Autodesk Inventor part; units mm, degrees
ref_plane "YZ Plane" through (0, 0, 0) normal (1, 0, 0) x (0, 1, 0)
ref_plane "XZ Plane" through (0, 0, 0) normal (0, 1, 0) x (-1, 0, 0)
ref_plane "XY Plane" through (0, 0, 0) normal (0, 0, 1) x (1, 0, 0)
sketch "Sketch1" plane through (0, 0, 0) normal (0, 1, 0) x (-1, 0, 0)
  line L0 (82.5, 55) -> (-82.5, 55)
  line L1 (-82.5, 55) -> (-82.5, -55)
  line L2 (-82.5, -55) -> (82.5, -55)
  line L3 (82.5, -55) -> (82.5, 55)
  line L4 (82.5, 55) -> (-82.5, -55) construction
  line L5 (-82.5, 55) -> (82.5, -55) construction
  point P0 (0, 0)
  dimension "d0" = 165
  dimension "d1" = 110
extrude "Extrusion1" add sketch "Sketch1" along normal blind 15
sketch "Sketch3" plane through (0, 15, 0) normal (0, 1, 0) x (1, 0, 0)
  line L0 (82.5, -55) -> (82.5, 55)
  line L1 (-82.5, -35.5) -> (82.5, -35.5)
  line L2 (82.5, -35.5) -> (82.5, 35.5)
  line L3 (82.5, 35.5) -> (-82.5, 35.5)
  line L4 (-82.5, 35.5) -> (-82.5, -35.5)
  line L5 (-82.5, -35.5) -> (82.5, 35.5) construction
  line L6 (82.5, -35.5) -> (-82.5, 35.5) construction
  point P0 (0, 0)
  dimension "d8" = 71
extrude "Extrusion3" cut sketch "Sketch3" against normal blind 5
sketch "Sketch4" plane through (0, 15, 0) normal (0, 1, 0) x (1, 0, 0)
  circle A0 centre (-67.5, -45) radius 4
  line L0 (-82.5, -55) -> (82.5, -55)
  line L1 (-82.5, -35.5) -> (-82.5, -55)
  line L2 (-82.5, -45) -> (82.5, -45)
  line L3 (82.5, -55) -> (82.5, 55)
  circle A1 centre (-27.5, -45) radius 4
  line L4 (-82.5, -55) -> (82.5, -55)
  line L5 (0, -55) -> (0, 55)
  line L6 (82.5, 55) -> (-82.5, 55)
  line L7 (-82.5, 55) -> (-82.5, -55)
  line L8 (-82.5, 0) -> (82.5, 0)
  circle A2 centre (67.5, -45) radius 4
  circle A3 centre (27.5, -45) radius 4
  circle A4 centre (-67.5, 45) radius 4
  circle A5 centre (-27.5, 45) radius 4
  circle A6 centre (67.5, 45) radius 4
  circle A7 centre (27.5, 45) radius 4
  point P0 (0, 0)
  dimension "d11" = 10
  dimension "d12" = 8
  dimension "d17" = 15
  dimension "d19" = 27.5
sketch "Sketch5" plane through (0, 10, 0) normal (0, 1, 0) x (1, 0, 0)
  line L0 (-52.5, -23) -> (52.5, -23)
  line L1 (52.5, -23) -> (52.5, 23)
  line L2 (52.5, 23) -> (-52.5, 23)
  line L3 (-52.5, 23) -> (-52.5, -23)
  line L4 (-52.5, -23) -> (52.5, 23) construction
  line L5 (52.5, -23) -> (-52.5, 23) construction
  line L6 (-82.5, 35.5) -> (82.5, 35.5)
  line L7 (-82.5, -35.5) -> (-82.5, 35.5)
  point P0 (0, 0)
  dimension "d13" = 12.5
  dimension "d14" = 30
extrude "Extrusion4" cut sketch "Sketch5" against normal through all
extrude "Extrusion5" cut sketch "Sketch4" against normal through all contours L2 A0 | A0 L2 | A1 L2 | L2 A1 | A3 L2 | L2 A3 | A2 L2 | L2 A2 | A4 | A5 | A6 | A7
sketch "Sketch6" plane through (0, 15, 0) normal (0, 1, 0) x (1, 0, 0)
  line L0 (-82.5, -55) -> (82.5, -55)
  line L1 (82.5, 55) -> (-82.5, 55)
  line L2 (-16.5, -55) -> (-2.5, -55)
  line L3 (-2.5, -55) -> (-2.5, 55)
  line L4 (-2.5, 55) -> (-16.5, 55)
  line L5 (-16.5, 55) -> (-16.5, -55)
  line L6 (82.5, -55) -> (82.5, -35.5)
  point P0 (0, 0)
  dimension "d22" = 85
  dimension "d23" = 14
extrude "Extrusion6" cut sketch "Sketch6" against normal up to surface (5 mm away)
properties part number "Clamps_v4_davidcell"
Input: part model. Units: mm. Frame: model coordinates. A direction names the side the tool comes from. Round coordinates to 2 decimals unless told otherwise and drop trailing zeros. Order: outer loops, then holes, each group sorted by start corner. A loop starts at its lowest first (then second) coordinate and runs counter-clockwise, first axis right, second up. Notation, with made-up numbers: (67.5, 47.5) - (79.5, 47.5) arc R27 cw to (79.5, 68.5) - close; hole circle Ø2 at (20, -2). An arc over 180 degrees is marked (long way). Use a Markdown table: item, result.
1. First-contact query: pin 1 (2 mm diameter, centred on x = -1, z = -23.5, fed in from +Y). Flat tip, straight axial feed; report the tip coordinate or a pass-through.
Evaluation:
| item | result |
|---|---|
| pin 1 | y = 10 |
2. Section D-D on x = 27.5. Return the cut outline in (y, z).
Evaluation:
| item | result |
|---|---|
| outline | (0, -55) - (15, -55) - (15, -49) - (0, -49) - close; (0, -41) - (15, -41) - (15, -35.5) - (10, -35.5) - (10, -23) - (0, -23) - close; (0, 23) - (10, 23) - (10, 35.5) - (15, 35.5) - (15, 41) - (0, 41) - close; (0, 49) - (15, 49) - (15, 55) - (0, 55) - close |
3. Section B-B on y = 12.75. State how many separate pieces and enclosed holes the cut face has, then the cut area to 3 significant figures.
Evaluation:
| item | result |
|---|---|
| separate pieces | 4 |
| enclosed holes | 8 |
| area | 5,490 mm^2 |
4. Material intervals for probe 1 along X at (y, z) = (6.75, 45); probe 2 along Z at (x, y) = (-27.5, 4.75); probe 3 along Z at (x, y) = (-67.5, 6.5), sorted ascending.
Evaluation:
| item | result |
|---|---|
| probe 1 | -82.5 to -71.5, -63.5 to -31.5, -23.5 to 23.5, 31.5 to 63.5, 71.5 to 82.5 |
| probe 2 | -55 to -49, -41 to -23, 23 to 41, 49 to 55 |
| probe 3 | -55 to -49, -41 to 41, 49 to 55 |
5. Access query for faces 5 (the face through (-16.5, 13, 45)), 6 (the face through (52.5, 5, 0)), 7 (the face through (41, 15, 45)), 8 (the face through (41, 13, -35.5)). Directions: +Z, -Z, +X, -X, +Y, -Y. A direction counts if a zero-diameter tool reaches every point of the face in a straight line with its end or side. Return the directions, or none.
Evaluation:
| item | result |
|---|---|
| face 5 | +Z, -Z, +Y |
| face 6 | +Y, -Y |
| face 7 | +Z, -Z, +X, -X, +Y |
| face 8 | +X, -X, +Y |
6. Mould query, pull axis X, two halves, no side actions, for faces 1 (the face through (1, 0, 25)), 2 (the face through (82.5, 6, 1)), 3 (the face through (-82.5, 6, -1)), 4 (the face through (-63.685, 7.605, 43.799)). Classes: +X half, -X half, draft (parallel to the pull), parting line (faces both ways), or undercut.
Evaluation:
| item | result |
|---|---|
| face 1 | draft |
| face 2 | +X half |
| face 3 | -X half |
| face 4 | undercut |
7. Section A-A on x = 67.5. Return the cut outline in (y, z).
Evaluation:
| item | result |
|---|---|
| outline | (0, -55) - (15, -55) - (15, -49) - (0, -49) - close; (0, -41) - (15, -41) - (15, -35.5) - (10, -35.5) - (10, 35.5) - (15, 35.5) - (15, 41) - (0, 41) - close; (0, 49) - (15, 49) - (15, 55) - (0, 55) - close |
8. Section C-C on z = 45. Return the cut outline in (x, y).
Evaluation:
| item | result |
|---|---|
| outline | (-82.5, 0) - (-71.5, 0) - (-71.5, 15) - (-82.5, 15) - close; (-63.5, 0) - (-31.5, 0) - (-31.5, 15) - (-63.5, 15) - close; (-23.5, 0) - (23.5, 0) - (23.5, 15) - (-2.5, 15) - (-2.5, 10) - (-16.5, 10) - (-16.5, 15) - (-23.5, 15) - close; (31.5, 0) - (63.5, 0) - (63.5, 15) - (31.5, 15) - close; (71.5, 0) - (82.5, 0) - (82.5, 15) - (71.5, 15) - close |
